Autodesk Inventor part; units mm, degrees
ref_plane "YZ Plane" through (0, 0, 0) normal (1, 0, 0) x (0, 1, 0)
ref_plane "XZ Plane" through (0, 0, 0) normal (0, 1, 0) x (-1, 0, 0)
ref_plane "XY Plane" through (0, 0, 0) normal (0, 0, 1) x (1, 0, 0)
sketch "Sketch1" plane through (0, 0, 0) normal (0, 0, 1) x (1, 0, 0)
  circle A0 centre (0, 0) radius 2.5
  circle A1 centre (0, 0) radius 4.5
  circle A2 centre (0, -10) radius 1.25
  circle A3 centre (0, -10) radius 3
  circle A4 centre (0, -10) radius 4
  circle A5 centre (0, 0) radius 1.25
  line L0 (-4.4944, -0.225) -> (-3.995, -10.2)
  line L1 (4.4944, -0.225) -> (3.995, -10.2)
  line L2 (0, 0) -> (0, -19.0302) construction
  point P0 (66.1895, -52.0583)
  point P1 (148.6808, -39.1685)
  point P2 (99.1548, -7.9801)
  point P3 (101.772, -8.3287)
  point P4 (96.5376, -8.3287)
  dimension "d8" = 9
  dimension "d13" = 5
  dimension "d25" = 2.5
  dimension "d26" = 6
  dimension "d27" = 8
  dimension "d28" = 2.5
  dimension "d29" = 10
extrude "Extrusion1" add sketch "Sketch1" along normal blind 0.5 contours A1 | A1 L1 A4 L0 | A4
extrude "Extrusion2" add sketch "Sketch1" along normal blind 2 contours A0 | A3
properties part number "ヘッケン抑え" material "アルミニウム 2014-T6"
The model under review builds one solid part; all positions refer to its coordinate system, in mm. A direction names the side the tool comes from. Give positions to 0.01 mm unless a question says otherwise; leave off trailing zeros. Write each loop counter-clockwise with the first axis right and the second up, starting at its lowest first coordinate (ties: lowest second). Pieces come first, ordered by that corner, then holes.
1. Draft analysis for pull direction X (two halves, no side actions). For faces 1 (the cylindrical face through (-0.16, -11.24, 0.99)), 2 (the cylindrical face through (-0.54, 2.44, 1.24)), 3 (the flat face through (1, 1, 2)), state which applies: +X half, -X half, draft (parallel to the pull), parting line (faces both ways), or undercut.
2. Wall thickness on L1, parallel to Y at x = 0, z = 1.1; L2, parallel to Y at x = 1, z = 1; L3, parallel to Z at x = 1.75, y = -6.75: over which ranges is each line inside the solid? List them lowest first.
3. Tool access review of faces 4 (the cylindrical face through (-3, -10, 1)), 5 (the cylindrical face through (-0.27, 1.22, 0.99)): name each direction out of +Z, -Z, +X, -X, +Y, -Y from which nothing blocks a thin tool from reaching the whole face with its end or side.
4. Add section D-D, the plane x = -2.25. Write out the cut boundary in (y, z).
5. Add section C-C, the plane z = 0.8. Write out the cut boundary in (x, y).
6. Add section B-B, the plane y = 0. Write out the cut boundary in (x, z).
7. For P1, Ø2, axis at x = 0, y = 0, coming from the +Z side; P2, Ø1, axis at y = 2, z = 1.5, coming from the +X side, all flat-tipped, find the tip position at first contact; note any pin that passes through.
8. Add section A-A, the plane x = 0. Write out the cut boundary in (y, z).
Worked answers:
1. face 1: undercut
1. face 2: parting line
1. face 3: draft
2. L1: y = -13 to -11.25, -8.75 to -7, -2.5 to -1.25, 1.25 to 2.5
2. L2: y = -12.83 to -10.75, -9.25 to -7.17, -2.29 to -0.75, 0.75 to 2.29
2. L3: z = 0 to 0.5
3. face 4: +Z
3. face 5: +Z, -Z
4. outline: (-13.31, 0) - (3.9, 0) - (3.9, 0.5) - (1.09, 0.5) - (1.09, 2) - (-1.09, 2) - (-1.09, 0.5) - (-8.02, 0.5) - (-8.02, 2) - (-11.98, 2) - (-11.98, 0.5) - (-13.31, 0.5) - close
5. outline: circle Ø6 at (0, -10); circle Ø5 at (0, 0); hole circle Ø2.5 at (0, -10); hole circle Ø2.5 at (0, 0)
6. outline: (-4.5, 0) - (-1.25, 0) - (-1.25, 2) - (-2.5, 2) - (-2.5, 0.5) - (-4.5, 0.5) - close; (1.25, 0) - (4.5, 0) - (4.5, 0.5) - (2.5, 0.5) - (2.5, 2) - (1.25, 2) - close
7. P1: passes through
7. P2: stops at x = 2
8. outline: (-14, 0) - (-11.25, 0) - (-11.25, 2) - (-13, 2) - (-13, 0.5) - (-14, 0.5) - close; (-8.75, 0) - (-1.25, 0) - (-1.25, 2) - (-2.5, 2) - (-2.5, 0.5) - (-7, 0.5) - (-7, 2) - (-8.75, 2) - close; (1.25, 0) - (4.5, 0) - (4.5, 0.5) - (2.5, 0.5) - (2.5, 2) - (1.25, 2) - close
